Read the model definition and answer for the solid it produces. Units are mm, in the model's axes. Coordinates: 2 decimals unless noted, no trailing zeros. Order: outer loops, then holes, each group sorted by start corner. A loop starts at its lowest first (then second) coordinate and runs counter-clockwise, first axis right, second up. Notation, with made-up numbers: (-14.5, 85) - (1.5, 85) arc R6 cw to (1.5, 95) - close; hole circle Ø10 at (35.25, 21). An arc over 180 degrees is marked (long way). Use one line per item in the form item = value. Start each with the question number.
from build123d import *

# Parameters (mm, degrees)
SKETCH1_W               = 48
SKETCH1_H               = 20
BOSS_EXTRUDE1_DEPTH     = 70
SKETCH3_R               = 4.15
CUT_EXTRUDE2_DEPTH      = 21
CUT_EXTRUDE3_DEPTH      = 1
CUT_EXTRUDE3_DEPTH_BACK = 71


with BuildPart() as part:
    # Sketch1 → Boss-Extrude1 (new body)
    with BuildSketch(Plane(origin=(0, 0, 0), x_dir=(1, 0, 0), z_dir=(0, 1, 0))):
        Rectangle(SKETCH1_W, SKETCH1_H)
    extrude(amount=BOSS_EXTRUDE1_DEPTH)

    # Sketch3 → Cut-Extrude2 (cut, through all)
    with BuildSketch(Plane.XY.offset(10)):
        with Locations((17, 53)):
            Circle(SKETCH3_R)
        with Locations((-17, 53)):
            Circle(SKETCH3_R)
        with Locations((-17, 17)):
            Circle(SKETCH3_R)
        with Locations((17, 17)):
            Circle(SKETCH3_R)
    extrude(amount=-CUT_EXTRUDE2_DEPTH, mode=Mode.SUBTRACT)

    # Sketch4 → Cut-Extrude3 (cut, two sides)
    with BuildSketch(Plane(origin=(0, 70, 0), x_dir=(1, 0, 0), z_dir=(0, 1, 0))) as cut_extrude3_sk:
        with BuildLine():
            Line((-7, 93.783466983), (-7, 10))
            ThreePointArc((-7, 10), (0, 3), (7, 10))
            Line((7, 10), (7, 93.783466983))
            Line((7, 93.783466983), (7, 261.350400948))
            Line((7, 261.350400948), (-7, 261.350400948))
            Line((-7, 261.350400948), (-7, 93.783466983))
        make_face()
    extrude(amount=CUT_EXTRUDE3_DEPTH, mode=Mode.SUBTRACT)
    extrude(cut_extrude3_sk.sketch, amount=-CUT_EXTRUDE3_DEPTH_BACK, mode=Mode.SUBTRACT)


solid = part.part
Q1. A cutting plane is placed at A-A (z = 0.25). Give the vertices of the cut face in (x, y), then the cut area to 3 significant figures.
Q2. A cutting plane is placed at B-B (y = 53). Give the vertices of the cut face in (x, z).
Q3. Consider probe 1 along Y at (x, z) = (17, 1.75); probe 2 along Y at (x, z) = (-20, 3); probe 3 along X at (y, z) = (49.5, -5.25). Determine where each line is inside the solid, lowest interval first.
Q4. For a pull along X with two mould halves and no side action, classify faces 1 (the flat face through (0, 70, 0)), 2 (the flat face through (24, 35, 0)), 3 (the cylindrical face through (-17.54, 57.115, 0.14)) as +X half, -X half, draft (parallel to the pull), parting line (faces both ways), or undercut.
Q5. A cutting plane is placed at C-C (x = 17). Give the vertices of the cut face in (y, z), then the cut area to 3 significant figures.
Q6. A cutting plane is placed at D-D (z = -7.5). Give the vertices of the cut face in (x, y), then the cut area to 3 significant figures.
Result sheet:
q1.outline = (-24, 0) - (24, 0) - (24, 70) - (-24, 70) - close; hole circle Ø8.3 at (-17, 17); hole circle Ø8.3 at (-17, 53); hole circle Ø8.3 at (17, 17); hole circle Ø8.3 at (17, 53)
q1.area = 3,140 mm^2
q2.outline = (-24, -10) - (-21.15, -10) - (-21.15, 10) - (-24, 10) - close; (-12.85, -10) - (-7, -10) arc R7 cw to (7, -10) - (12.85, -10) - (12.85, 10) - (-12.85, 10) - close; (21.15, -10) - (24, -10) - (24, 10) - (21.15, 10) - close
q3.probe_1 = 0 to 12.85, 21.15 to 48.85, 57.15 to 70
q3.probe_2 = 0 to 14.13, 19.87 to 50.13, 55.87 to 70
q3.probe_3 = -24 to -19.23, -14.77 to -5.14, 5.14 to 14.77, 19.23 to 24
q4.face_1 = draft
q4.face_2 = +X half
q4.face_3 = undercut
q5.outline = (0, -10) - (12.85, -10) - (12.85, 10) - (0, 10) - close; (21.15, -10) - (48.85, -10) - (48.85, 10) - (21.15, 10) - close; (57.15, -10) - (70, -10) - (70, 10) - (57.15, 10) - close
q5.area = 1,070 mm^2
q6.outline = (-24, 0) - (-6.54, 0) - (-6.54, 70) - (-24, 70) - close; (6.54, 0) - (24, 0) - (24, 70) - (6.54, 70) - close; hole circle Ø8.3 at (-17, 17); hole circle Ø8.3 at (-17, 53); hole circle Ø8.3 at (17, 17); hole circle Ø8.3 at (17, 53)
q6.area = 2,230 mm^2
